For this review, take the finished solid that the model builds, in its own axes (mm). Face numbers are marked on the shaded views. Coordinates: 2 decimals unless noted, no trailing zeros. Write each loop counter-clockwise with the first axis right and the second up, starting at its lowest first coordinate (ties: lowest second). Pieces come first, ordered by that corner, then holes. Notation, with made-up numbers: M 44,-2 L 83,-2 A21 cw 83,32 Z; hole C -2,74.25 d9. An arc over 180 degrees is marked long. Return JSON: item names as keys, results as strings.
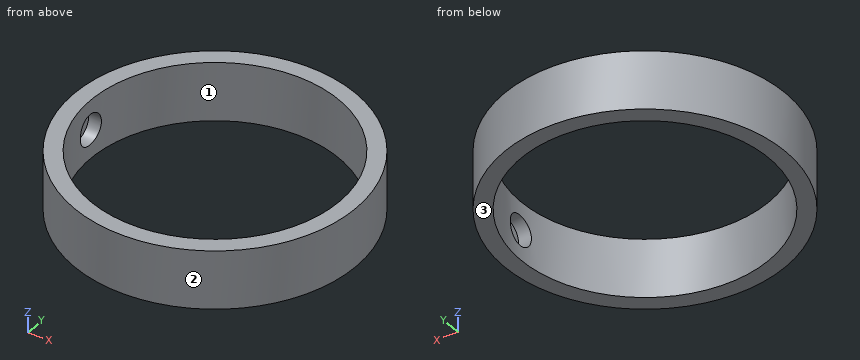
```python
from build123d import *

# Parameters (mm, degrees)
F0_R          = 15.24
F0_R_2        = 13.462
F1_DEPTH      = 3.175
F2_R          = 1.651
F3_DEPTH      = 14.732
F3_DEPTH_BACK = 14.732


with BuildPart() as f1:
    # F0 (on Top) → F1 (new body, symmetric)
    with BuildSketch(Plane.XY):
        Circle(F0_R)
        Circle(F0_R_2, mode=Mode.SUBTRACT)
    extrude(amount=F1_DEPTH, both=True)

    # F2 (on Right) → F3 (cut, two sides)
    with BuildSketch(Plane.YZ) as f3_sk:
        Circle(F2_R)
    extrude(amount=-F3_DEPTH, mode=Mode.SUBTRACT)
    extrude(f3_sk.sketch, amount=F3_DEPTH_BACK, mode=Mode.SUBTRACT)


solid = f1.part
```
1. Draft analysis for pull direction X (two halves, no side actions). For the marked faces 1, 2 and 3, state which applies: +X half, -X half, draft (parallel to the pull), parting line (faces both ways), or undercut.
Checks:
{"face 1": "undercut", "face 2": "parting line", "face 3": "draft"}
2. We need section C-C (x = -10.5). State the section outline as (y, z) points (3 decimals), plus the area to 3 significant figures.
Checks:
{"outline": "M -11.046,-3.175 L -8.425,-3.175 L -8.425,3.175 L -11.046,3.175 Z; M 8.425,-3.175 L 11.046,-3.175 L 11.046,3.175 L 8.425,3.175 Z", "area": "33.3 mm2"}
3. We need section A-A (z = 0). State the section outline as (x, y) points.
Checks:
{"outline": "C 0,0 d30.48; hole M -14.73,-1.65 L -13.36,-1.65 A13.46 ccw 13.36,-1.65 L 14.73,-1.65 L 14.73,1.65 L 13.36,1.65 A13.46 ccw -13.36,1.65 L -14.73,1.65 Z"}
4. We need section B-B (y = 0). State the section outline as (x, z) points (3 decimals).
Checks:
{"outline": "M -15.24,-3.175 L -13.462,-3.175 L -13.462,-1.651 L -14.732,-1.651 L -14.732,1.651 L -13.462,1.651 L -13.462,3.175 L -15.24,3.175 Z; M 13.462,-3.175 L 15.24,-3.175 L 15.24,3.175 L 13.462,3.175 L 13.462,1.651 L 14.732,1.651 L 14.732,-1.651 L 13.462,-1.651 Z"}
5. Wall thickness on L1, parallel to Z at x = 14.35, y = 0 (3 decimals); L2, parallel to X at y = 1.5, z = 1.75; L3, parallel to Y at x = 8, z = 2: over which ranges is each line inside the solid? List them lowest first. Write a range as from..to.
Checks:
{"L1": "-3.175..-1.651, 1.651..3.175", "L2": "-15.17..-13.38, 13.38..15.17", "L3": "-12.97..-10.83, 10.83..12.97"}
6. Clearance check with flat-ended pins moving along their axes: pin 1 Ø3 at (x, z) = (-4, 0.5) entering from +Y; pin 2 Ø16 at (x, y) = (0, 0) entering from +Z; pin 3 Ø2.5 at (y, z) = (0.5, -1) entering from -X; pin 4 Ø2 at (x, z) = (8, -1) entering from +Y. State where each tip first meets the part, or that it passes through.
Checks:
{"pin 1": "y = 15.03", "pin 2": "through", "pin 3": "x = -15.24", "pin 4": "y = 13.54"}
